Print and shaded views of the part. All mm, measured from the part's lowest x, y and z. A direction names the side the tool comes from. Coordinates: 2 decimals unless noted, no trailing zeros. Order: outer loops, then holes, each group sorted by start corner. A loop starts at its lowest first (then second) coordinate and runs counter-clockwise, first axis right, second up. Notation, with made-up numbers: (60.25, 32.5) -> (102.25, 32.5) arc R16 ccw to (102.25, 60.5) -> close; hole circle Ø3 at (62, -17.75). An arc over 180 degrees is marked (long way). Return JSON: item names as keys, results as strings. Group by question number.
1) Cut at C-C (z = 76). Write the cut outline in (x, y).
2) Cut at A-A (x = 8.5). Write the cut outline in (y, z).
3) Flat gauge pins, fed straight in: pin 1 (18 mm diameter, centred on x = 20.65, z = 50.11, fed in from -Y); pin 2 (12 mm diameter, centred on x = 26.5, y = 28.5, fed in from +Z); pin 3 (12 mm diameter, centred on x = 26.5, y = 35.5, fed in from -Z). Where does each tip first touch, or does it go through?
4) Probe line 1 (Y direction, x = 16, z = 66); line 2 (Y direction, x = 7.5, z = 37.5); line 3 (Z direction, x = 36.5, y = 26.5). List the from-to ranges inside material, lowest first.
5) Pull direction Y, two halves, no side cores. Call the marked faces 4, 5, 6 and 7: +Y half, -Y half, draft (parallel to the pull), parting line (faces both ways), or undercut.
6) Cut at D-D (y = 25). Write the cut outline in (x, z), and give its area (3 significant figures).
7) Cut at B-B (y = 49.5). Write the cut outline in (x, z).
8) Which spindle directions (+Z, -Z, +X, -X, +Y, -Y) get a long thin tool onto all of the face, cutting with end or side? Do the marked faces 1, 2 and 3. Say none if no direction does.
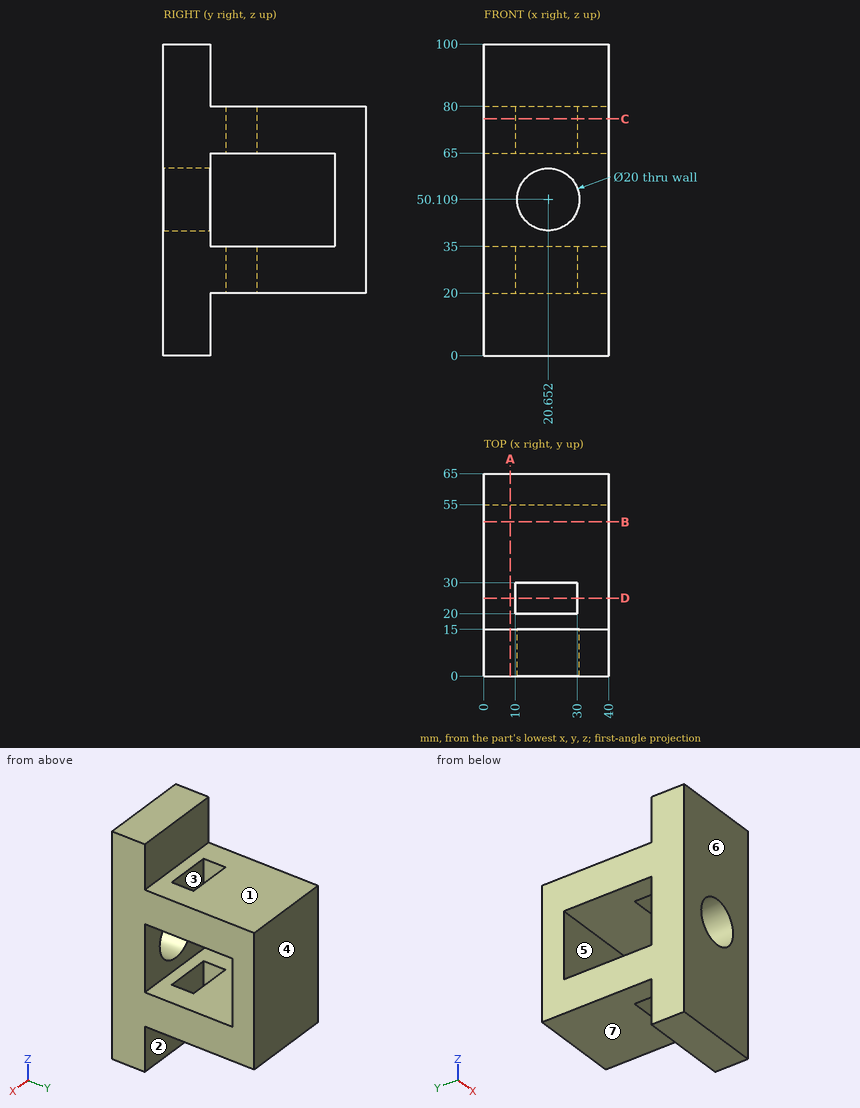
Answers below:
{
 "1": {"outline": "(0, 0) -> (40, 0) -> (40, 65) -> (0, 65) -> close; hole (10, 20) -> (30, 20) -> (30, 30) -> (10, 30) -> close"},
 "2": {"outline": "(0, 0) -> (15, 0) -> (15, 20) -> (65, 20) -> (65, 80) -> (15, 80) -> (15, 100) -> (0, 100) -> close; hole (15, 35) -> (55, 35) -> (55, 65) -> (15, 65) -> close"},
 "3": {"pin 1": "stops at y = 55", "pin 2": "stops at z = 80", "pin 3": "stops at z = 20"},
 "4": {"line 1": "y = 0 to 20, 30 to 65", "line 2": "y = 0 to 15, 55 to 65", "line 3": "z = 20 to 35, 65 to 80"},
 "5": {"face 4": "+Y half", "face 5": "undercut", "face 6": "-Y half", "face 7": "draft"},
 "6": {"outline": "(0, 20) -> (10, 20) -> (10, 35) -> (0, 35) -> close; (0, 65) -> (10, 65) -> (10, 80) -> (0, 80) -> close; (30, 20) -> (40, 20) -> (40, 35) -> (30, 35) -> close; (30, 65) -> (40, 65) -> (40, 80) -> (30, 80) -> close", "area": "600 mm^2"},
 "7": {"outline": "(0, 20) -> (40, 20) -> (40, 35) -> (0, 35) -> close; (0, 65) -> (40, 65) -> (40, 80) -> (0, 80) -> close"},
 "8": {"face 1": "+Z, +X, -X, +Y", "face 2": "-Z, +X, -X, +Y", "face 3": "+Z, -Z"}
}
